Part model, mm, in its own coordinate system. Round coordinates to 2 decimals unless told otherwise and drop trailing zeros. Order: outer loops, then holes, each group sorted by start corner. A loop starts at its lowest first (then second) coordinate and runs counter-clockwise, first axis right, second up. Notation, with made-up numbers: M 12.25,24.25 L 64.25,24.25 A12 cw 64.25,29.25 Z; hole C -5,-2.5 d8. An arc over 180 degrees is marked long. Write each question's results on one line, items separated by ' | '. Start each with the question number.
1. Probe L1, parallel to X at y = -16.2, z = 0; L2, parallel to Y at x = -21.5, z = 0 (3 decimals); L3, parallel to Z at x = -53, y = 11.5. List the from-to ranges inside material, lowest first. Write a range as [from, to].
2. Band-saw the part on C-C, the plane y = 8. List the corners of the cut face in (x, z).
3. Band-saw the part on B-B, the plane x = -27. List the corners of the cut face in (y, z) (3 decimals).
4. Band-saw the part on A-A, the plane z = 0. List the corners of the cut face in (x, y) (3 decimals).
5. Band-saw the part on D-D, the plane z = 14.5. List the corners of the cut face in (x, y), then the cut area to 3 significant figures.
6. Drop flat-ended pins along their axis: pin 1 Ø3 at (x, z) = (-21, -2.5) entering from +Y; pin 2 Ø8 at (x, y) = (-44, 6) entering from -Z; pin 3 Ø10.5 at (x, z) = (-58.86, 0) entering from +Y. Give the stop position or say it passes through.
7. Two-plate mould, pull along Z, no slides. Class faces 1 (the face through (-38.63, -17.24, 17.14)), 2 (the face through (0, -17, 1)), 3 (the face through (-53.41, 16.91, 1.72)): +Z half, -Z half, draft (parallel to the pull), parting line (faces both ways), or undercut.
```python
from build123d import *

# Parameters (mm, degrees)
BASE_EXTRUDE_DEPTH = 76.2
SKETCH3_R          = 15.875
CUT_EXTRUDE2_DEPTH = 81.82230509
SKETCH2_R          = 5.715
CUT_EXTRUDE1_DEPTH = 88.298066989
FILLET1_R          = 6.35


with BuildPart() as part:
    # Sketch1 → Base-Extrude (new body)
    with BuildSketch(Plane(origin=(0, 0, 0), x_dir=(0, 0, -1), z_dir=(1, 0, 0))):
        with BuildLine():
            Line((19.05, 0), (19.05, -19.05))
            Line((19.05, -19.05), (-19.05, -19.05))
            Line((-19.05, -19.05), (-19.05, 0))
            ThreePointArc((-19.05, 0), (0, 19.05), (19.05, 0))
        make_face()
    extrude(amount=-BASE_EXTRUDE_DEPTH)

    # Sketch3 → Cut-Extrude2 (cut, through all)
    with BuildSketch(Plane(origin=(0, 0, 0), x_dir=(0, 0, -1), z_dir=(1, 0, 0))):
        Circle(SKETCH3_R)
    extrude(amount=-CUT_EXTRUDE2_DEPTH, mode=Mode.SUBTRACT)

    # Sketch2 → Cut-Extrude1 (cut, through all)
    with BuildSketch(Plane.XZ.offset(19.05)):
        with Locations((-14.409818925, 0)):
            Circle(SKETCH2_R)
        with Locations((-58.859818925, 0)):
            Circle(SKETCH2_R)
    extrude(amount=-CUT_EXTRUDE1_DEPTH, mode=Mode.SUBTRACT)

    # Fillet1
    fillet1_edges = [part.edges().sort_by_distance(p)[0] for p in [
        (-38.1, -19.05, 19.05),
        (-38.1, -19.05, -19.05),
    ]]
    fillet(fillet1_edges, radius=FILLET1_R)


solid = part.part
```
Solution:
1) L1: [-76.2, -64.57], [-53.14, -20.12], [-8.69, 0] | L2: [-19.05, -15.875], [15.875, 19.05] | L3: [-15.19, -10.94], [10.94, 15.19]
2) outline: M -76.2,-17.29 L 0,-17.29 L 0,-13.71 L -76.2,-13.71 Z; M -76.2,13.71 L 0,13.71 L 0,17.29 L -76.2,17.29 Z
3) outline: M -19.05,-12.7 A6.35 ccw -12.7,-19.05 L 0,-19.05 A19.05 ccw 0,19.05 L -12.7,19.05 A6.35 ccw -19.05,12.7 Z; hole C 0,0 d31.75
4) outline: M -76.2,-19.05 L -64.575,-19.05 L -64.575,-15.875 L -76.2,-15.875 Z; M -76.2,15.875 L -64.575,15.875 L -64.575,19.05 L -76.2,19.05 Z; M -53.145,-19.05 L -20.125,-19.05 L -20.125,-15.875 L -53.145,-15.875 Z; M -53.145,15.875 L -20.125,15.875 L -20.125,19.05 L -53.145,19.05 Z; M -8.695,-19.05 L 0,-19.05 L 0,-15.875 L -8.695,-15.875 Z; M -8.695,15.875 L 0,15.875 L 0,19.05 L -8.695,19.05 Z
5) outline: M -76.2,-18.79 L 0,-18.79 L 0,-6.46 L -76.2,-6.46 Z; M -76.2,6.46 L 0,6.46 L 0,12.36 L -76.2,12.36 Z | area: 1,390 mm^2
6) pin 1: y = 19.02 | pin 2: z = -18.94 | pin 3: through
7) face 1: +Z half | face 2: draft | face 3: undercut
